Work out the finished part from the listing and answer in its coordinate system (mm). Round coordinates to 2 decimals unless told otherwise and drop trailing zeros. Write each loop counter-clockwise with the first axis right and the second up, starting at its lowest first coordinate (ties: lowest second). Pieces come first, ordered by that corner, then holes. Notation, with made-up numbers: M -3.5,-37.5 L 10.5,-37.5 A21 cw 10.5,-14.5 Z; hole C 13,45.25 d11. An arc over 180 degrees is marked long. One line per item, written item: value. Start each with the question number.
Q1. Find section B-B (x = 35). Write down the section's boundary in (y, z), and give its area (3 significant figures).
Q2. Find section D-D (y = 3). Write down the section's boundary in (x, z), and give its area (3 significant figures).
Q3. Given pin 1 Ø0.9 at (y, z) = (37.5, 2) entering from -X; pin 2 Ø1.8 at (x, z) = (4, 1) entering from +Y, each flat-ended and moving along its own axis, determine where each tip first touches the part or whether it passes through.
Q4. Find section A-A (y = 20.5). Write down the section's boundary in (x, z).
Q5. Find section C-C (x = 43.4). Write down the section's boundary in (y, z), and give its area (3 significant figures).
Q6. Consider probe 1 along Y at (x, z) = (43.4, 0.7); probe 2 along X at (y, z) = (26.5, 1.95); probe 3 along Y at (x, z) = (39, 1.8). Determine where each line is inside the solid, lowest interval first.
from build123d import *

# Parameters (mm, degrees)
ESBO_O1_W                = 48
ESBO_O1_H                = 40
RESSALTO_EXTRUS_O1_DEPTH = 3
ESBO_O2_R                = 1
CORTE_EXTRUS_O1_DEPTH    = 4
ESBO_O3_W                = 9.79419224
ESBO_O3_H                = 12.19966749
ESBO_O3_H_2              = 11.54056128
ESBO_O3_W_2              = 8.914185242
CORTE_EXTRUS_O2_DEPTH    = 10
CORTE_EXTRUS_O3_DEPTH    = 4
ESBO_O5_R                = 1
ESBO_O5_R_2              = 0.998470841
CORTE_EXTRUS_O4_DEPTH    = 4


with BuildPart() as part:
    # Esboço1 → Ressalto-extrusão1 (new body)
    with BuildSketch(Plane.XY):
        with Locations((26.7, 20)):
            Rectangle(ESBO_O1_W, ESBO_O1_H)
    extrude(amount=RESSALTO_EXTRUS_O1_DEPTH)

    # Esboço2 → Corte-extrusão1 (cut, through all)
    with BuildSketch(Plane.XY.offset(3)):
        with Locations((10, 37)):
            Circle(ESBO_O2_R)
        with Locations((10, 3)):
            Circle(ESBO_O2_R)
        with Locations((43.4, 3)):
            Circle(ESBO_O2_R)
        with Locations((43.4, 37)):
            Circle(ESBO_O2_R)
    extrude(amount=-CORTE_EXTRUS_O1_DEPTH, mode=Mode.SUBTRACT)

    # Esboço3 → Corte-extrusão2 (cut)
    with BuildSketch(Plane.XY.offset(3)):
        with Locations((53.2961889, 40.797789277)):
            Rectangle(ESBO_O3_W, ESBO_O3_H)
        with Locations((53.2961889, -0.072325108)):
            Rectangle(ESBO_O3_W, ESBO_O3_H_2)
        with Locations((0.54181876, -0.072325108)):
            Rectangle(ESBO_O3_W_2, ESBO_O3_H_2)
        with Locations((0.54181876, 40.797789277)):
            Rectangle(ESBO_O3_W_2, ESBO_O3_H)
    extrude(amount=-CORTE_EXTRUS_O2_DEPTH, mode=Mode.SUBTRACT)

    # Esboço4 → Corte-extrusão3 (cut, through all)
    with BuildSketch(Plane.XY.offset(3)):
        Polygon((8.956927741, 31.209698911), (6.956927741, 29.209698911), (6.956927741, 11.209698911), (8.956927741, 9.209698911), (43.956927741, 9.209698911), (45.956927741, 11.209698911), (45.956927741, 29.209698911), (43.956927741, 31.209698911), align=None)
    extrude(amount=-CORTE_EXTRUS_O3_DEPTH, mode=Mode.SUBTRACT)

    # Esboço5 → Corte-extrusão4 (cut, through all)
    with BuildSketch(Plane.XY.offset(3)):
        with Locations((5.956927741, 31.709698911)):
            Circle(ESBO_O5_R)
        with Locations((46.956927741, 31.709698911)):
            Circle(ESBO_O5_R_2)
        with Locations((46.956927741, 8.709698911)):
            Circle(ESBO_O5_R)
        with Locations((5.956927741, 8.709698911)):
            Circle(ESBO_O5_R)
    extrude(amount=-CORTE_EXTRUS_O4_DEPTH, mode=Mode.SUBTRACT)


solid = part.part
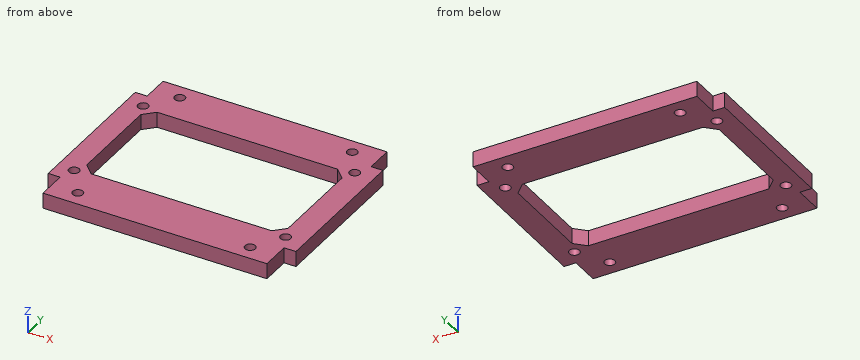
The answers:
1. outline: M 0,0 L 9.21,0 L 9.21,3 L 0,3 Z; M 31.21,0 L 40,0 L 40,3 L 31.21,3 Z
1. area: 54.0 mm2
2. outline: M 5,0 L 9,0 L 9,3 L 5,3 Z; M 11,0 L 42.4,0 L 42.4,3 L 11,3 Z; M 44.4,0 L 48.4,0 L 48.4,3 L 44.4,3 Z
2. area: 118 mm2
3. pin 1: x = 5
3. pin 2: y = 34.7
4. outline: M 2.7,0 L 6.96,0 L 6.96,3 L 2.7,3 Z; M 45.96,0 L 50.7,0 L 50.7,3 L 45.96,3 Z
5. outline: M 0,0 L 2,0 L 2,3 L 0,3 Z; M 4,0 L 9.21,0 L 9.21,3 L 4,3 Z; M 31.21,0 L 36,0 L 36,3 L 31.21,3 Z; M 38,0 L 40,0 L 40,3 L 38,3 Z
5. area: 42.0 mm2
6. probe 1: 0 to 2, 4 to 9.21, 31.21 to 36, 38 to 40
6. probe 2: 2.7 to 6.96, 45.96 to 50.7
6. probe 3: 0 to 9.21, 31.21 to 40
